from build123d import *

# Parameters (mm, degrees)
SKETCH1_W                = 30
SKETCH1_H                = 4
BOSS_EXTRUDE1_DEPTH      = 7
SKETCH2_W                = 1.9
SKETCH2_H                = 1.9
BOSS_EXTRUDE2_DEPTH      = 1
SKETCH3_W                = 1.9
SKETCH3_H                = 1.769397694
BOSS_EXTRUDE3_DEPTH      = 1
BOSS_EXTRUDE3_DEPTH_BACK = 1
SKETCH4_R                = 0.519223145
SKETCH4_R_2              = 0.583770961
SKETCH4_R_3              = 0.581603631
CUT_EXTRUDE2_DEPTH       = 1
CUT_EXTRUDE2_DEPTH_BACK  = 3


with BuildPart() as part:
    # Sketch1 → Boss-Extrude1 (new body)
    with BuildSketch(Plane(origin=(0, 0, 0), x_dir=(0, 0, -1), z_dir=(1, 0, 0))):
        with Locations((15, 2)):
            Rectangle(SKETCH1_W, SKETCH1_H)
    extrude(amount=BOSS_EXTRUDE1_DEPTH)

    # Sketch2 → Boss-Extrude2 (add)
    with BuildSketch(Plane(origin=(0, 0, 0), x_dir=(0, 0, -1), z_dir=(1, 0, 0))):
        with Locations((5.150612861, 2.196174594)):
            Rectangle(SKETCH2_W, SKETCH2_H)
    extrude(amount=-BOSS_EXTRUDE2_DEPTH)

    # Sketch3 → Boss-Extrude3 (add, two sides)
    with BuildSketch(Plane(origin=(0, 0, 0), x_dir=(0, 0, -1), z_dir=(1, 0, 0))) as boss_extrude3_sk:
        with Locations((24.756915523, 2.019063583)):
            Rectangle(SKETCH3_W, SKETCH3_H)
    extrude(amount=BOSS_EXTRUDE3_DEPTH)
    extrude(boss_extrude3_sk.sketch, amount=-BOSS_EXTRUDE3_DEPTH_BACK)

    # Sketch4 → Cut-Extrude2 (cut, two sides)
    with BuildSketch(Plane(origin=(7, 0, 0), x_dir=(0, 0, -1), z_dir=(1, 0, 0))) as cut_extrude2_sk:
        with Locations((7.5, 2)):
            Circle(SKETCH4_R)
        with Locations((15, 2)):
            Circle(SKETCH4_R_2)
        with Locations((22.508486169, 2)):
            Circle(SKETCH4_R_3)
    extrude(amount=CUT_EXTRUDE2_DEPTH, mode=Mode.SUBTRACT)
    extrude(cut_extrude2_sk.sketch, amount=-CUT_EXTRUDE2_DEPTH_BACK, mode=Mode.SUBTRACT)


solid = part.part
Could you check a few things on this model? Use its own coordinates, in mm. A direction names the side the tool comes from. Give positions to 0.01 mm unless a question says otherwise; leave off trailing zeros. Write each loop counter-clockwise with the first axis right and the second up, starting at its lowest first coordinate (ties: lowest second). Pieces come first, ordered by that corner, then holes. Notation, with made-up numbers: (-2, -7.5) -> (52, -7.5) arc R17 ccw to (52, 0.5) -> close; hole circle Ø2 at (-12, 43). An arc over 180 degrees is marked (long way). Answer as CSV lines item,"result". Start each with the question number.
(1) If we mould it in two halves opening along Z, with no side actions, what happens to faces 5 (the face through (-0.5, 2, -25.707)), 6 (the face through (-0.5, 3.146, -5.1)), 7 (the face through (5.521, 2.175, -15.557))? For each: +Z half, -Z half, draft (parallel to the pull), parting line (faces both ways), or undercut.
(2) I'm going to push flat-ended pins straight in: pin 1 Ø2 at (y, z) = (1.5, -16.5) entering from -X; pin 2 Ø0.8 at (x, y) = (-0.5, 2.5) entering from +Z; pin 3 Ø0.8 at (y, z) = (2, -7.5) entering from +X. Where does each tip first touch, or does it pass through?
(3) If we section it at D-D, the plane z = -7.5: Write out the boundary of the cut face in (x, y).
(4) If we section it at C-C, the plane y = 2: Write out the boundary of the cut face in (x, z), and give its area (3 significant figures).
(5) If we section it at B-B, the plane z = -15: Write out the boundary of the cut face in (x, y), and give its area (3 significant figures).
(6) Which directions (+Z, -Z, +X, -X, +Y, -Y) give clear straight access to the entire face, cutting with the end or side of a thin tool? Please do faces 1 (the face through (-0.5, 2, -23.807)), 2 (the face through (4, 2, -7.5)), 3 (the face through (-0.5, 2.2, -4.201)), 4 (the face through (-0.5, 2.904, -24.7)).
(7) If we section it at A-A, the plane x = 4.5: Write out the boundary of the cut face in (y, z).
(8) Please list where these lines run through material, in increasing order: line 1 (Z direction, x = 5, y = 1.95); line 2 (Y direction, x = 4.65, z = -7.5); line 3 (Y direction, x = 6.35, z = -15).
Answer list:
1,face 5,"-Z half"
1,face 6,"draft"
1,face 7,"undercut"
2,pin 1,"x = 0"
2,pin 2,"z = -4.2"
2,pin 3,"x = 4"
3,outline,"(0, 0) -> (7, 0) -> (7, 1.48) -> (4, 1.48) -> (4, 2.52) -> (7, 2.52) -> (7, 4) -> (0, 4) -> close"
4,outline,"(-1, -25.71) -> (0, -25.71) -> (0, -30) -> (7, -30) -> (7, -23.09) -> (4, -23.09) -> (4, -21.93) -> (7, -21.93) -> (7, -15.58) -> (4, -15.58) -> (4, -14.42) -> (7, -14.42) -> (7, -8.02) -> (4, -8.02) -> (4, -6.98) -> (7, -6.98) -> (7, 0) -> (0, 0) -> (0, -4.2) -> (-1, -4.2) -> (-1, -6.1) -> (0, -6.1) -> (0, -23.81) -> (-1, -23.81) -> close"
4,area,"204 mm^2"
5,outline,"(0, 0) -> (7, 0) -> (7, 1.42) -> (4, 1.42) -> (4, 2.58) -> (7, 2.58) -> (7, 4) -> (0, 4) -> close"
5,area,"24.5 mm^2"
6,face 1,"-X, +Y, -Y"
6,face 2,"+X"
6,face 3,"+Z, -X, +Y, -Y"
6,face 4,"-Z, -X, +Y"
7,outline,"(0, -30) -> (4, -30) -> (4, 0) -> (0, 0) -> close; hole circle Ø1.16 at (2, -22.51); hole circle Ø1.17 at (2, -15); hole circle Ø1.04 at (2, -7.5)"
8,line 1,"-30 to -23.09, -21.93 to -15.58, -14.42 to -8.02, -6.98 to 0"
8,line 2,"0 to 1.48, 2.52 to 4"
8,line 3,"0 to 1.42, 2.58 to 4"
